Source: three-view drawing plus pictorial views. Frame: mm from the lowest corner of the part. Coordinates: 2 decimals unless noted, no trailing zeros. Order: outer loops, then holes, each group sorted by start corner. A loop starts at its lowest first (then second) coordinate and runs counter-clockwise, first axis right, second up. Notation, with made-up numbers: (25, -31.5) - (69, -31.5) arc R23 cw to (69, -5.5) - close; hole circle Ø9 at (-29, 32.25). An arc over 180 degrees is marked (long way). One line per question, with ' | ' between items.
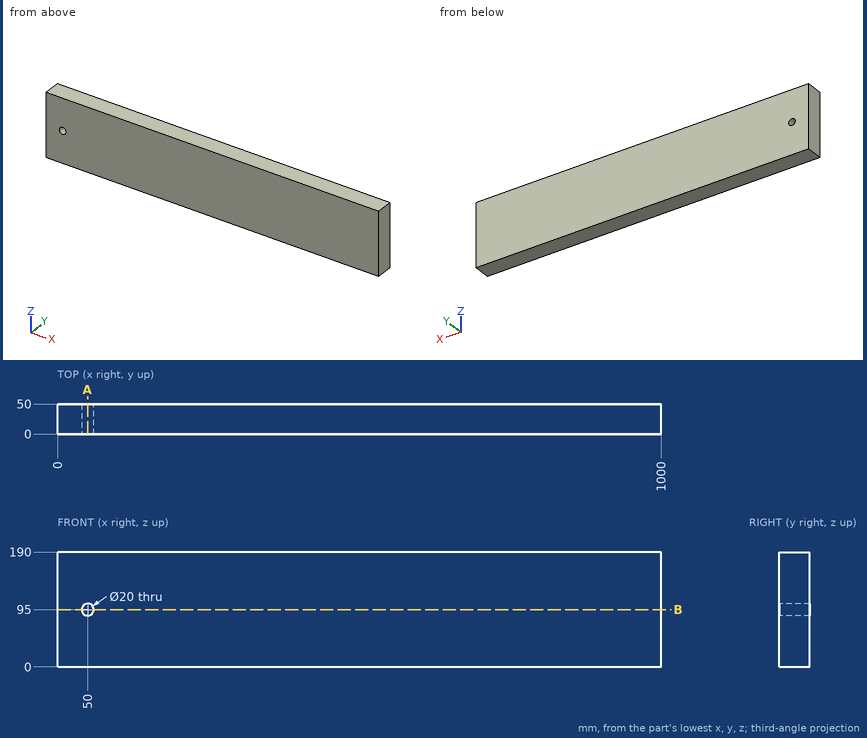
Item 1: Ray query, line 1 (Z direction, x = 50, y = 16); line 2 (X direction, y = 38, z = 99.5). Return the intervals inside material, ascending.
Data:
line 1: 0 to 85, 105 to 190 | line 2: 0 to 41.07, 58.93 to 1000
Item 2: Section A-A on x = 50. Return the cut outline in (y, z), and give its area (3 significant figures).
Data:
outline: (0, 0) - (50, 0) - (50, 85) - (0, 85) - close; (0, 105) - (50, 105) - (50, 190) - (0, 190) - close | area: 8,500 mm^2
Item 3: Section B-B on z = 95. Return the cut outline in (x, y).
Data:
outline: (0, 0) - (40, 0) - (40, 50) - (0, 50) - close; (60, 0) - (1000, 0) - (1000, 50) - (60, 50) - close
